Source: CAD feature listing. Evaluate the final solid. Frame: model axes, mm. A direction names the side the tool comes from. Give positions to 0.01 mm unless a question says otherwise; leave off trailing zeros. Write each loop counter-clockwise with the first axis right and the second up, starting at its lowest first coordinate (ties: lowest second). Pieces come first, ordered by that corner, then holes. Notation, with made-up numbers: (65.25, 82) -> (100.25, 82) arc R20 ccw to (100.25, 107) -> close; hole circle Ø6 at (6, 53.25). An arc over 180 degrees is marked (long way). Answer as a JSON object with one key per item and string values. Group by question number.
Item 1: Access query for faces 4 (the face through (38, 59, 0.1)), 5 (the face through (93.9, 30, 3)), 6 (the face through (26, 59, -1.7)). Directions: +Z, -Z, +X, -X, +Y, -Y. A direction counts if a zero-diameter tool reaches every point of the face in a straight line with its end or side. Return the directions, or none.
Item 2: Section query C-C on x = 82. Return the cut outline in (y, z).
Item 3: First-contact query: pin 1 Ø2 at (y, z) = (49.5, 4) entering from +X; pin 2 Ø1.5 at (x, y) = (28.5, 23) entering from +Z; pin 3 Ø1.6 at (x, y) = (49, 59) entering from +Z. Flat tips, straight axial feed; report the tip coordinate or a pass-through.
Item 4: Section query A-A on x = 95.75. Return the cut outline in (y, z), plus the area to 3 significant figures.
Item 5: Ray query, probe 1 along Y at (x, z) = (22.95, -0.65); probe 2 along Z at (x, y) = (55, 52.5); probe 3 along Z at (x, y) = (25, 19.5). Return the intervals inside material, ascending. Write a range as from..to.
Item 6: Pull-direction query (Y, two-part tool) for faces 1 (the face through (2.1, 1.3, -0.8)), 2 (the face through (38, 59, -1.7)), 3 (the face through (50, 60.3, -1)); classes: pulls with the +Y half, pulls with the -Y half, needs draft (parallel to the pull), parting line crosses it, or undercut.
Item 7: Section query D-D on z = 3.5. Return the cut outline in (x, y), plus the area to 3 significant figures.
Item 8: Section query B-B on y = 50. Return the cut outline in (x, z), plus the area to 3 significant figures.
from build123d import *

# Parameters (mm, degrees)
SKETCH1_W                = 98.5
SKETCH1_H                = 60.3
BOSS_EXTRUDE1_DEPTH      = 1.6
F_3_0_3_DIAMETER_HOLE1_D = 3
SKETCH5_W                = 89.3
SKETCH5_H                = 41.8
BOSS_EXTRUDE2_DEPTH      = 5.4
SKETCH6_W                = 76
SKETCH6_H                = 25.2
CUT_EXTRUDE1_DEPTH       = 0.5
BOSS_EXTRUDE3_DEPTH      = 0.1
BOSS_EXTRUDE3_DEPTH_BACK = 1.7
F_1_0_1_DIAMETER_HOLE1_D = 1


with BuildPart() as part:
    # Sketch1 → Boss-Extrude1 (new body)
    with BuildSketch(Plane.XY):
        with Locations((49.25, 30.15)):
            Rectangle(SKETCH1_W, SKETCH1_H)
    extrude(amount=-BOSS_EXTRUDE1_DEPTH)

    # Ø3.0 (3) Diameter Hole1 (through all)
    with Locations(Plane.XY):
        with Locations((2.75, 57.65), (95.75, 57.65), (95.75, 2.65), (2.75, 2.65)):
            Hole(F_3_0_3_DIAMETER_HOLE1_D / 2)

    # Sketch5 → Boss-Extrude2 (add)
    with BuildSketch(Plane.XY):
        with Locations((49.25, 30.15)):
            Rectangle(SKETCH5_W, SKETCH5_H)
    extrude(amount=BOSS_EXTRUDE2_DEPTH)

    # Sketch6 → Cut-Extrude1 (cut)
    with BuildSketch(Plane.XY.offset(5.4)):
        with Locations((49.25, 30.15)):
            Rectangle(SKETCH6_W, SKETCH6_H)
    extrude(amount=-CUT_EXTRUDE1_DEPTH, mode=Mode.SUBTRACT)

    # Sketch7 → Boss-Extrude3 (add, two sides: drawn at the far end of the back side and taken through both)
    with BuildSketch(Plane(origin=(0, 0, -1.6), x_dir=(-1, 0, 0), z_dir=(0, 0, -1)).offset(-BOSS_EXTRUDE3_DEPTH_BACK)):
        with BuildLine():
            Line((-11.25, 58.15), (-11.25, 60.3))
            Line((-11.25, 60.3), (-9.25, 60.3))
            Line((-9.25, 60.3), (-9.25, 58.15))
            ThreePointArc((-9.25, 58.15), (-10.25, 57.15), (-11.25, 58.15))
        make_face()
        with BuildLine():
            Line((-11.79, 58.15), (-11.79, 60.3))
            Line((-11.79, 60.3), (-13.79, 60.3))
            Line((-13.79, 60.3), (-13.79, 58.15))
            ThreePointArc((-13.79, 58.15), (-12.79, 57.15), (-11.79, 58.15))
        make_face()
        with BuildLine():
            Line((-14.33, 58.15), (-14.33, 60.3))
            Line((-14.33, 60.3), (-16.33, 60.3))
            Line((-16.33, 60.3), (-16.33, 58.15))
            ThreePointArc((-16.33, 58.15), (-15.33, 57.15), (-14.33, 58.15))
        make_face()
        with BuildLine():
            Line((-16.87, 58.15), (-16.87, 60.3))
            Line((-16.87, 60.3), (-18.87, 60.3))
            Line((-18.87, 60.3), (-18.87, 58.15))
            ThreePointArc((-18.87, 58.15), (-17.87, 57.15), (-16.87, 58.15))
        make_face()
        with BuildLine():
            Line((-19.41, 58.15), (-19.41, 60.3))
            Line((-19.41, 60.3), (-21.41, 60.3))
            Line((-21.41, 60.3), (-21.41, 58.15))
            ThreePointArc((-21.41, 58.15), (-20.41, 57.15), (-19.41, 58.15))
        make_face()
        with BuildLine():
            Line((-21.95, 58.15), (-21.95, 60.3))
            Line((-21.95, 60.3), (-23.95, 60.3))
            Line((-23.95, 60.3), (-23.95, 58.15))
            ThreePointArc((-23.95, 58.15), (-22.95, 57.15), (-21.95, 58.15))
        make_face()
        with BuildLine():
            Line((-24.49, 58.15), (-24.49, 60.3))
            Line((-24.49, 60.3), (-26.49, 60.3))
            Line((-26.49, 60.3), (-26.49, 58.15))
            ThreePointArc((-26.49, 58.15), (-25.49, 57.15), (-24.49, 58.15))
        make_face()
        with BuildLine():
            Line((-27.03, 58.15), (-27.03, 60.3))
            Line((-27.03, 60.3), (-29.03, 60.3))
            Line((-29.03, 60.3), (-29.03, 58.15))
            ThreePointArc((-29.03, 58.15), (-28.03, 57.15), (-27.03, 58.15))
        make_face()
        with BuildLine():
            Line((-29.57, 58.15), (-29.57, 60.3))
            Line((-29.57, 60.3), (-31.57, 60.3))
            Line((-31.57, 60.3), (-31.57, 58.15))
            ThreePointArc((-31.57, 58.15), (-30.57, 57.15), (-29.57, 58.15))
        make_face()
        with BuildLine():
            Line((-32.11, 58.15), (-32.11, 60.3))
            Line((-32.11, 60.3), (-34.11, 60.3))
            Line((-34.11, 60.3), (-34.11, 58.15))
            ThreePointArc((-34.11, 58.15), (-33.11, 57.15), (-32.11, 58.15))
        make_face()
        with BuildLine():
            Line((-34.65, 58.15), (-34.65, 60.3))
            Line((-34.65, 60.3), (-36.65, 60.3))
            Line((-36.65, 60.3), (-36.65, 58.15))
            ThreePointArc((-36.65, 58.15), (-35.65, 57.15), (-34.65, 58.15))
        make_face()
        with BuildLine():
            Line((-37.19, 58.15), (-37.19, 60.3))
            Line((-37.19, 60.3), (-39.19, 60.3))
            Line((-39.19, 60.3), (-39.19, 58.15))
            ThreePointArc((-39.19, 58.15), (-38.19, 57.15), (-37.19, 58.15))
        make_face()
        with BuildLine():
            Line((-39.73, 58.15), (-39.73, 60.3))
            Line((-39.73, 60.3), (-41.73, 60.3))
            Line((-41.73, 60.3), (-41.73, 58.15))
            ThreePointArc((-41.73, 58.15), (-40.73, 57.15), (-39.73, 58.15))
        make_face()
        with BuildLine():
            Line((-42.27, 58.15), (-42.27, 60.3))
            Line((-42.27, 60.3), (-44.27, 60.3))
            Line((-44.27, 60.3), (-44.27, 58.15))
            ThreePointArc((-44.27, 58.15), (-43.27, 57.15), (-42.27, 58.15))
        make_face()
        with BuildLine():
            Line((-44.81, 58.15), (-44.81, 60.3))
            Line((-44.81, 60.3), (-46.81, 60.3))
            Line((-46.81, 60.3), (-46.81, 58.15))
            ThreePointArc((-46.81, 58.15), (-45.81, 57.15), (-44.81, 58.15))
        make_face()
        with BuildLine():
            Line((-47.35, 58.15), (-47.35, 60.3))
            Line((-47.35, 60.3), (-49.35, 60.3))
            Line((-49.35, 60.3), (-49.35, 58.15))
            ThreePointArc((-49.35, 58.15), (-48.35, 57.15), (-47.35, 58.15))
        make_face()
    extrude(amount=BOSS_EXTRUDE3_DEPTH + BOSS_EXTRUDE3_DEPTH_BACK)

    # Ø1.0 (1) Diameter Hole1 (through all)
    with Locations(Plane.XY.offset(0.1)):
        with Locations((10.25, 58.15), (12.79, 58.15), (15.33, 58.15), (17.87, 58.15), (20.41, 58.15), (22.95, 58.15), (25.49, 58.15), (28.03, 58.15), (30.57, 58.15), (33.11, 58.15), (35.65, 58.15), (38.19, 58.15), (40.73, 58.15), (43.27, 58.15), (45.81, 58.15), (48.35, 58.15)):
            Hole(F_1_0_1_DIAMETER_HOLE1_D / 2)


solid = part.part
Worked answers:
{
 "1": {"face 4": "+Z, +X, -X, +Y", "face 5": "+Z, +X, +Y, -Y", "face 6": "-Z, +X, -X, +Y, -Y"},
 "2": {"outline": "(0, -1.6) -> (60.3, -1.6) -> (60.3, 0) -> (51.05, 0) -> (51.05, 5.4) -> (42.75, 5.4) -> (42.75, 4.9) -> (17.55, 4.9) -> (17.55, 5.4) -> (9.25, 5.4) -> (9.25, 0) -> (0, 0) -> close"},
 "3": {"pin 1": "x = 93.9", "pin 2": "z = 4.9", "pin 3": "z = 0.1"},
 "4": {"outline": "(0, -1.6) -> (1.15, -1.6) -> (1.15, 0) -> (0, 0) -> close; (4.15, -1.6) -> (56.15, -1.6) -> (56.15, 0) -> (4.15, 0) -> close; (59.15, -1.6) -> (60.3, -1.6) -> (60.3, 0) -> (59.15, 0) -> close", "area": "86.9 mm^2"},
 "5": {"probe 1": "0..57.65, 58.65..60.3", "probe 2": "-1.6..0", "probe 3": "-1.6..4.9"},
 "6": {"face 1": "undercut", "face 2": "needs draft", "face 3": "pulls with the +Y half"},
 "7": {"outline": "(4.6, 9.25) -> (93.9, 9.25) -> (93.9, 51.05) -> (4.6, 51.05) -> close", "area": "3,730 mm^2"},
 "8": {"outline": "(0, -1.6) -> (98.5, -1.6) -> (98.5, 0) -> (93.9, 0) -> (93.9, 5.4) -> (4.6, 5.4) -> (4.6, 0) -> (0, 0) -> close", "area": "640 mm^2"}
}
